Drawing for the job (mm, zero at the part's lowest x, y, z). A direction names the side the tool comes from. Give positions to 0.01 mm unless a question says otherwise; leave off trailing zeros. Loops run counter-clockwise (first coordinate to the right, second up) from the corner with the lowest first, then second, coordinate; pieces in that order, holes last.
1) 3-axis set-ups, long thin cutter, end or side, ignore diameter. For the marked faces 1 and 2: which of +Z, -Z, +X, -X, +Y, -Y reach the whole face in a straight line?
2) Band-saw the part on A-A on z = 19.85. List the corners of the cut face in (x, y), then the cut area to 3 significant figures.
3) Wall check: line 1 (X direction, y = 4.3, z = 19.85); line 2 (Z direction, x = 20.4, y = 3.15); line 3 (Z direction, x = 22.5, y = 5.1). Give the ranges that are in metal, low to high.
4) Band-saw the part on D-D on z = 32. List the corners of the cut face in (x, y), then the cut area to 3 significant figures.
5) Flat gauge pin, fed straight in: P1, Ø18, axis at x = 28.5, z = 21.5, coming from the -Y side. Where does the tip first touch, or does it go through?
6) Band-saw the part on B-B on x = 11.5. List the corners of the cut face in (y, z).
7) Band-saw the part on C-C on y = 4.95. List the corners of the cut face in (x, z), then the cut area to 3 significant figures.
8) Two-plate mould, pull along X, no slides. Class the marked faces 3, 4, 5 and 6: +X half, -X half, draft (parallel to the pull), parting line (faces both ways), or undercut.
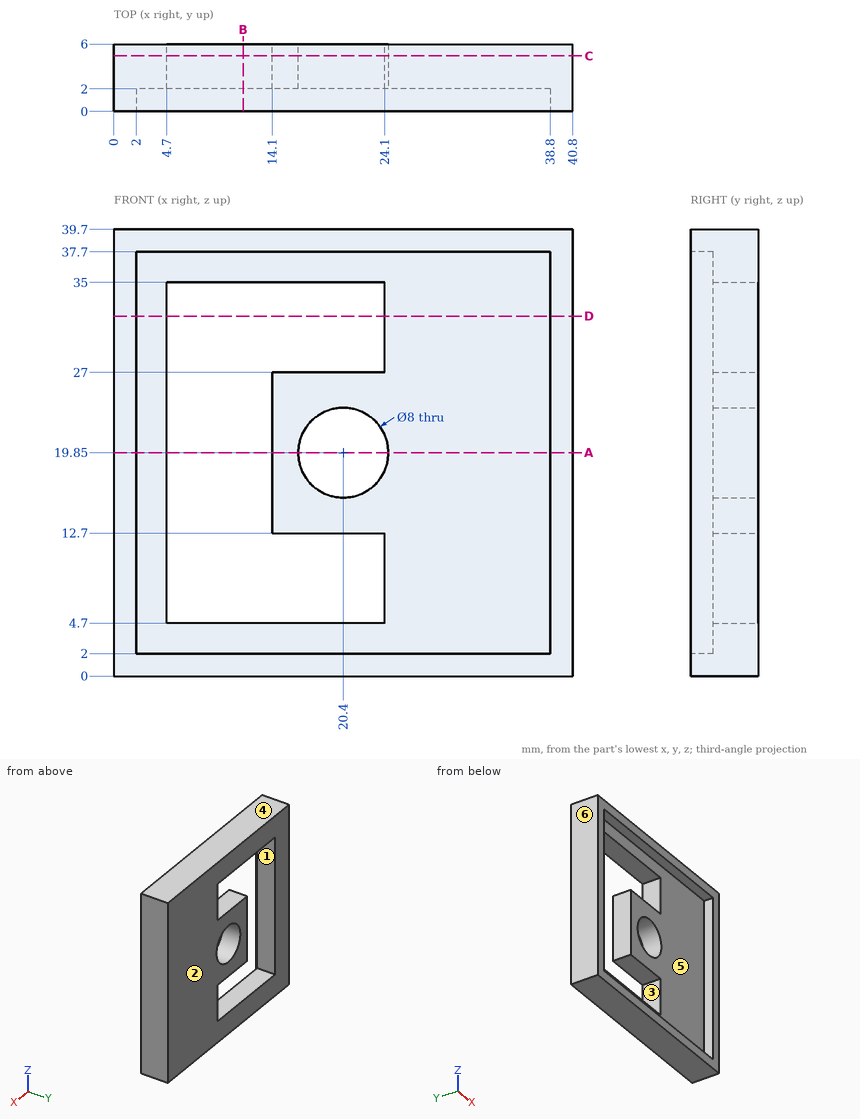
Findings below:
1. face 1: +Y, -Y
1. face 2: +Z, -Z, +X, -X, +Y
2. outline: (0, 0) - (2, 0) - (2, 2) - (4.7, 2) - (4.7, 6) - (0, 6) - close; (14.1, 2) - (16.4, 2) - (16.4, 6) - (14.1, 6) - close; (24.4, 2) - (38.8, 2) - (38.8, 0) - (40.8, 0) - (40.8, 6) - (24.4, 6) - close
2. area: 102 mm2
3. line 1: x = 0 to 4.7, 14.1 to 16.4, 24.4 to 40.8
3. line 2: z = 0 to 4.7, 12.7 to 15.85, 23.85 to 27, 35 to 39.7
3. line 3: z = 0 to 4.7, 12.7 to 16.45, 23.25 to 27, 35 to 39.7
4. outline: (0, 0) - (2, 0) - (2, 2) - (4.7, 2) - (4.7, 6) - (0, 6) - close; (24.1, 2) - (38.8, 2) - (38.8, 0) - (40.8, 0) - (40.8, 6) - (24.1, 6) - close
4. area: 93.6 mm2
5. P1: stops at y = 2
6. outline: (0, 0) - (6, 0) - (6, 4.7) - (2, 4.7) - (2, 2) - (0, 2) - close; (0, 37.7) - (2, 37.7) - (2, 35) - (6, 35) - (6, 39.7) - (0, 39.7) - close
7. outline: (0, 0) - (40.8, 0) - (40.8, 39.7) - (0, 39.7) - close; hole (4.7, 4.7) - (24.1, 4.7) - (24.1, 12.7) - (14.1, 12.7) - (14.1, 27) - (24.1, 27) - (24.1, 35) - (4.7, 35) - close; hole circle Ø8 at (20.4, 19.85)
7. area: 1,120 mm2
8. face 3: undercut
8. face 4: draft
8. face 5: undercut
8. face 6: -X half
